Read the model definition and answer for the solid it produces. Units are mm, in the model's axes. A direction names the side the tool comes from. Coordinates: 2 decimals unless noted, no trailing zeros. Write each loop counter-clockwise with the first axis right and the second up, starting at its lowest first coordinate (ties: lowest second). Pieces come first, ordered by that corner, then holes. Notation, with made-up numbers: (39, 19) -> (64, 19) arc R6 ccw to (64, 24) -> close; hole circle Ø7 at (42.25, 45). An arc over 180 degrees is marked (long way). Answer as a JSON object with one key per item and string values. Group by question number.
(1) Which of the six approach directions +Z, -Z, +X, -X, +Y, -Y give full straight-line access (tool end or side, diameter ignored) to faces 4 (the face through (0.2, 3.5, 6.5)), 5 (the face through (-0.2, 0.5, 6.5)), 6 (the face through (11.956, 1.979, 0.984))?
(2) Flat-ended cylindrical pins translate along their axes: P1, Ø4, axis at x = -1.5, z = -6.5, coming from the +Y side; P2, Ø10, axis at x = -5.5, z = 0, coming from the -Y side; P3, Ø1, axis at y = 2, z = -8.5, coming from the +X side. Find the tip coordinate at first contact, or state that the pin passes through.
(3) Find section C-C (x = -9). Give the vertices of the cut face in (y, z), then the cut area to 3 significant figures.
(4) For a pull along Z with two mould halves and no side action, classify faces 1 (the face through (-7, 1.98, -0.33)), 2 (the face through (5.53, 2.22, 17.55)), 3 (the face through (-14, 4.5, -7)) as +Z half, -Z half, draft (parallel to the pull), parting line (faces both ways), or undercut.
(5) Find section A-A (x = 0). Give the vertices of the cut face in (y, z), then the cut area to 3 significant figures.
(6) Straight lines are drawn through the part: L1, parallel to X at y = 1.4, z = 0; L2, parallel to X at y = 4.05, z = 0; L3, parallel to Y at x = -6, z = -9.5. For each, find the intervals that lie inside material, in ascending order.
(7) Find section B-B (z = -2.5). Give the vertices of the cut face in (x, y), then the cut area to 3 significant figures.
(8) Find section D-D (z = 6.5). Give the vertices of the cut face in (x, y), then the cut area to 3 significant figures.
from build123d import *

# Parameters (mm, degrees)
SKETCH1_R           = 18.4
BOSS_EXTRUDE1_DEPTH = 4.5
SKETCH2_R           = 15
CUT_EXTRUDE1_DEPTH  = 1
SKETCH3_R           = 2.5
CUT_EXTRUDE2_DEPTH  = 27.40776401
CUT_EXTRUDE3_START  = -0.5
SKETCH4_R           = 15
CUT_EXTRUDE3_DEPTH  = 0.5
SKETCH5_R           = 6
CUT_EXTRUDE4_DEPTH  = 27.25585649


with BuildPart() as part:
    # Sketch1 → Boss-Extrude1 (new body)
    with BuildSketch(Plane(origin=(0, 0, 0), x_dir=(1, 0, 0), z_dir=(0, 1, 0))):
        with Locations(Location((0, 0, 0), (0, 0, 270))):
            Circle(SKETCH1_R)
    extrude(amount=BOSS_EXTRUDE1_DEPTH)

    # Sketch2 → Cut-Extrude1 (cut)
    with BuildSketch(Plane(origin=(0, 4.5, 0), x_dir=(1, 0, 0), z_dir=(0, 1, 0))):
        with Locations(Location((0, 0, 0), (0, 0, 270))):
            Circle(SKETCH2_R)
    extrude(amount=-CUT_EXTRUDE1_DEPTH, mode=Mode.SUBTRACT)

    # Sketch3 → Cut-Extrude2 (cut, through all)
    with BuildSketch(Plane.XZ):
        with Locations(Location((-9.477141659, -0.658624302, 0), (0, 0, 270))):
            Circle(SKETCH3_R)
        with Locations(Location((9.477141659, 0.658624302, 0), (0, 0, 270))):
            Circle(SKETCH3_R)
    extrude(amount=-CUT_EXTRUDE2_DEPTH, mode=Mode.SUBTRACT)

    # Sketch4 → Cut-Extrude3 (cut)
    with BuildSketch(Plane.XZ.offset(CUT_EXTRUDE3_START)):
        with Locations(Location((0, 0, 0), (0, 0, 90))):
            Circle(SKETCH4_R)
    extrude(amount=CUT_EXTRUDE3_DEPTH, mode=Mode.SUBTRACT)

    # Sketch5 → Cut-Extrude4 (cut, through all)
    with BuildSketch(Plane(origin=(0, 3.5, 0), x_dir=(1, 0, 0), z_dir=(0, 1, 0))):
        with Locations(Location((0, 0, 0), (0, 0, 270))):
            Circle(SKETCH5_R)
    extrude(amount=-CUT_EXTRUDE4_DEPTH, mode=Mode.SUBTRACT)


solid = part.part
Results below:
{
 "1": {"face 4": "+Y", "face 5": "-Y", "face 6": "+Y, -Y"},
 "2": {"P1": "stops at y = 3.5", "P2": "stops at y = 0.5", "P3": "stops at x = 16.57"},
 "3": {"outline": "(0, -16.05) -> (4.5, -16.05) -> (4.5, -12) -> (3.5, -12) -> (3.5, -3.11) -> (0.5, -3.11) -> (0.5, -12) -> (0, -12) -> close; (0, 12) -> (0.5, 12) -> (0.5, 1.8) -> (3.5, 1.8) -> (3.5, 12) -> (4.5, 12) -> (4.5, 16.05) -> (0, 16.05) -> close", "area": "93.7 mm2"},
 "4": {"face 1": "undercut", "face 2": "parting line", "face 3": "draft"},
 "5": {"outline": "(0, -18.4) -> (4.5, -18.4) -> (4.5, -15) -> (3.5, -15) -> (3.5, -6) -> (0.5, -6) -> (0.5, -15) -> (0, -15) -> close; (0, 15) -> (0.5, 15) -> (0.5, 6) -> (3.5, 6) -> (3.5, 15) -> (4.5, 15) -> (4.5, 18.4) -> (0, 18.4) -> close", "area": "84.6 mm2"},
 "6": {"L1": "x = -18.4 to -11.89, -7.07 to -6, 6 to 7.07, 11.89 to 18.4", "L2": "x = -18.4 to -15, 15 to 18.4", "L3": "y = 0.5 to 3.5"},
 "7": {"outline": "(-18.23, 0) -> (-14.79, 0) -> (-14.79, 0.5) -> (-11.17, 0.5) -> (-11.17, 3.5) -> (-14.79, 3.5) -> (-14.79, 4.5) -> (-18.23, 4.5) -> close; (-7.79, 0.5) -> (-5.45, 0.5) -> (-5.45, 3.5) -> (-7.79, 3.5) -> close; (5.45, 0.5) -> (14.79, 0.5) -> (14.79, 0) -> (18.23, 0) -> (18.23, 4.5) -> (14.79, 4.5) -> (14.79, 3.5) -> (5.45, 3.5) -> close", "area": "76.8 mm2"},
 "8": {"outline": "(-17.21, 0) -> (-13.52, 0) -> (-13.52, 0.5) -> (13.52, 0.5) -> (13.52, 0) -> (17.21, 0) -> (17.21, 4.5) -> (13.52, 4.5) -> (13.52, 3.5) -> (-13.52, 3.5) -> (-13.52, 4.5) -> (-17.21, 4.5) -> close", "area": "114 mm2"}
}
